Can you work these out from the model? Positions are in its coordinate system, mm. Give positions to 0.01 mm unless a question says otherwise; leave off trailing zeros. Order: outer loops, then holes, each group sorted by start corner. A loop starts at its lowest first (then second) coordinate and runs counter-clockwise, first axis right, second up. Notation, with made-up numbers: (7.25, -32.5) - (44.25, -32.5) arc R28 ccw to (44.25, -8.5) - close; hole circle Ø7 at (-30.75, 63). An arc over 180 degrees is marked (long way). Answer as CSV lines item,"result".
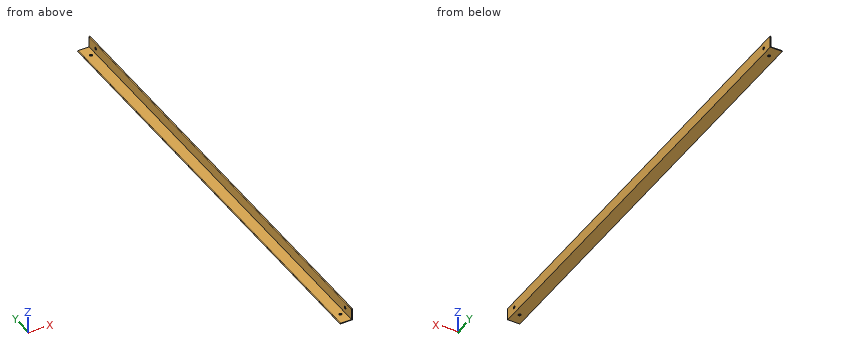
```python
from build123d import *

# Parameters (mm, degrees)
EXTRUDE_1_DEPTH        = 2000
FILLET_1_R             = 0.1
SKETCH_2_R             = 6
CUT_EXTRUDE_1_DEPTH    = 200
SKETCH_5_R             = 6
CUT_EXTRUDE_2_DEPTH    = 200
PATTERN_LINEAR_1_COUNT = 2
PATTERN_LINEAR_1_PITCH = 1900


with BuildPart() as part:
    # 草图1 → 凸台-拉伸1 (new body)
    with BuildSketch(Plane(origin=(0, 0, 0), x_dir=(1, 0, 0), z_dir=(0, 1, 0))):
        with BuildLine():
            ThreePointArc((-29.759542218, 3), (-28.958115236, 0.95539927), (-26.980771162, 0))
            Line((-26.980771162, 0), (-26.520700364, 0))
            Line((-26.520700364, 0), (20.240457782, 0))
            Line((20.240457782, 0), (20.240457782, -46.555391571))
            ThreePointArc((20.240457782, -46.555391571), (21.249360232, -48.99109755), (23.68506621, -50))
            Line((23.68506621, -50), (23.68506621, 3))
            Line((23.68506621, 3), (-29.759542218, 3))
        make_face()
    extrude(amount=EXTRUDE_1_DEPTH)

    # 圆角1
    # the kernel refuses this fillet: 0.1 mm, written as the material it takes off along each edge
    with BuildSketch(Plane(origin=(24.28506621, 2000, -3), x_dir=(0, 0, 1), z_dir=(-1, 0, 0))) as fillet_1_piece_1:
        with BuildLine():
            CenterArc((FILLET_1_R, -FILLET_1_R), FILLET_1_R, 90, 90)
            Line((0, -FILLET_1_R), (-FILLET_1_R * 0.02, -FILLET_1_R))
            Line((-FILLET_1_R * 0.02, -FILLET_1_R), (-FILLET_1_R * 0.02, FILLET_1_R * 0.0199999999995))
            Line((-FILLET_1_R * 0.02, FILLET_1_R * 0.0199999999995), (FILLET_1_R, FILLET_1_R * 0.0199999999995))
            Line((FILLET_1_R, FILLET_1_R * 0.0199999999995), (FILLET_1_R, 0))
        make_face()
    extrude(amount=54.644608429, mode=Mode.SUBTRACT)
    with BuildSketch(Plane(origin=(20.240457782, 2000, 0), x_dir=(0, 0, -1), z_dir=(-1, 0, 0)), Plane(origin=(-27.580771162, 0, 0), x_dir=(0, 0, -1), z_dir=(1, 0, 0))) as fillet_1_piece_2:
        with BuildLine():
            CenterArc((FILLET_1_R, FILLET_1_R), FILLET_1_R, 180, 90)
            Line((0, FILLET_1_R), (-FILLET_1_R * 0.02, FILLET_1_R))
            Line((-FILLET_1_R * 0.02, FILLET_1_R), (-FILLET_1_R * 0.02, -FILLET_1_R * 0.0199999999995))
            Line((-FILLET_1_R * 0.02, -FILLET_1_R * 0.0199999999995), (FILLET_1_R, -FILLET_1_R * 0.0199999999995))
            Line((FILLET_1_R, -FILLET_1_R * 0.0199999999995), (FILLET_1_R, 0))
        make_face()
    extrude(amount=47.821228944, mode=Mode.SUBTRACT)
    with BuildSketch(Plane(origin=(20.240457782, 2000, 0), x_dir=(1, 0, 0), z_dir=(0, 0, 1)), Plane(origin=(20.240457782, 0, 0), x_dir=(0, 1, 0), z_dir=(0, 0, 1))) as fillet_1_piece_3:
        with BuildLine():
            CenterArc((FILLET_1_R, -FILLET_1_R), FILLET_1_R, 90, 90)
            Line((0, -FILLET_1_R), (-FILLET_1_R * 0.02, -FILLET_1_R))
            Line((-FILLET_1_R * 0.02, -FILLET_1_R), (-FILLET_1_R * 0.02, FILLET_1_R * 0.0199999999995))
            Line((-FILLET_1_R * 0.02, FILLET_1_R * 0.0199999999995), (FILLET_1_R, FILLET_1_R * 0.0199999999995))
            Line((FILLET_1_R, FILLET_1_R * 0.0199999999995), (FILLET_1_R, 0))
        make_face()
    extrude(amount=46.555391571, mode=Mode.SUBTRACT)
    with BuildSketch(Plane(origin=(23.68506621, 2000, 46.555391571), x_dir=(-1, 0, 0), z_dir=(0, 0, -1))) as fillet_1_piece_4:
        with BuildLine():
            CenterArc((3.444608429 - FILLET_1_R, -FILLET_1_R), FILLET_1_R, 0, 90)
            Line((3.444608429, -FILLET_1_R), (3.444608429 + FILLET_1_R * 0.02, -FILLET_1_R))
            Line((3.444608429 + FILLET_1_R * 0.02, -FILLET_1_R), (3.444608429 + FILLET_1_R * 0.02, FILLET_1_R * 0.0199999999995))
            Line((3.444608429 + FILLET_1_R * 0.02, FILLET_1_R * 0.0199999999995), (3.444608429 - FILLET_1_R, FILLET_1_R * 0.0199999999995))
            Line((3.444608429 - FILLET_1_R, FILLET_1_R * 0.0199999999995), (3.444608429 - FILLET_1_R, 0))
        make_face()
    revolve(axis=Axis((23.68506621, 2000, 46.555391571), (0, 1, 0)), revolution_arc=99.984089086, mode=Mode.SUBTRACT)
    with BuildSketch(Plane(origin=(24.28506621, 0, -3), x_dir=(0, 0, 1), z_dir=(-1, 0, 0))) as fillet_1_piece_5:
        with BuildLine():
            CenterArc((FILLET_1_R, FILLET_1_R), FILLET_1_R, 180, 90)
            Line((0, FILLET_1_R), (-FILLET_1_R * 0.02, FILLET_1_R))
            Line((-FILLET_1_R * 0.02, FILLET_1_R), (-FILLET_1_R * 0.02, -FILLET_1_R * 0.02))
            Line((-FILLET_1_R * 0.02, -FILLET_1_R * 0.02), (FILLET_1_R, -FILLET_1_R * 0.02))
            Line((FILLET_1_R, -FILLET_1_R * 0.02), (FILLET_1_R, 0))
        make_face()
    extrude(amount=54.644608429, mode=Mode.SUBTRACT)
    with BuildSketch(Plane(origin=(23.68506621, 2000, 50.6), x_dir=(-1, 0, 0), z_dir=(0, 0, -1)), Plane(origin=(23.68506621, 0, 50.6), x_dir=(0, 1, 0), z_dir=(0, 0, -1))) as fillet_1_piece_6:
        with BuildLine():
            CenterArc((FILLET_1_R, -FILLET_1_R), FILLET_1_R, 90, 90)
            Line((0, -FILLET_1_R), (-FILLET_1_R * 0.02, -FILLET_1_R))
            Line((-FILLET_1_R * 0.02, -FILLET_1_R), (-FILLET_1_R * 0.02, FILLET_1_R * 0.0199999999995))
            Line((-FILLET_1_R * 0.02, FILLET_1_R * 0.0199999999995), (FILLET_1_R, FILLET_1_R * 0.0199999999995))
            Line((FILLET_1_R, FILLET_1_R * 0.0199999999995), (FILLET_1_R, 0))
        make_face()
    extrude(amount=54.2, mode=Mode.SUBTRACT)
    with BuildSketch(Plane(origin=(23.68506621, 0, 46.555391571), x_dir=(-1, 0, 0), z_dir=(0, 0, -1))) as fillet_1_piece_7:
        with BuildLine():
            CenterArc((3.444608429 - FILLET_1_R, FILLET_1_R), FILLET_1_R, 270, 90)
            Line((3.444608429 - FILLET_1_R, 0), (3.444608429 - FILLET_1_R, -FILLET_1_R * 0.02))
            Line((3.444608429 - FILLET_1_R, -FILLET_1_R * 0.02), (3.444608429 + FILLET_1_R * 0.02, -FILLET_1_R * 0.02))
            Line((3.444608429 + FILLET_1_R * 0.02, -FILLET_1_R * 0.02), (3.444608429 + FILLET_1_R * 0.02, FILLET_1_R))
            Line((3.444608429 + FILLET_1_R * 0.02, FILLET_1_R), (3.444608429, FILLET_1_R))
        make_face()
    revolve(axis=Axis((23.68506621, 0, 46.555391571), (0, 1, 0)), revolution_arc=99.984089086, mode=Mode.SUBTRACT)
    with BuildSketch(Plane(origin=(20.840457782, 2000, 0), x_dir=(0, 0, -1), z_dir=(-1, 0, 0))) as fillet_1_piece_8a_section:
        with BuildLine():
            CenterArc((FILLET_1_R, FILLET_1_R), FILLET_1_R, 180, 90)
            Line((0, FILLET_1_R), (-FILLET_1_R * 0.02, FILLET_1_R))
            Line((-FILLET_1_R * 0.02, FILLET_1_R), (-FILLET_1_R * 0.02, -FILLET_1_R * 0.0199999999995))
            Line((-FILLET_1_R * 0.02, -FILLET_1_R * 0.0199999999995), (FILLET_1_R, -FILLET_1_R * 0.0199999999995))
            Line((FILLET_1_R, -FILLET_1_R * 0.0199999999995), (FILLET_1_R, 0))
        make_face()
    fillet_1_piece_8a = extrude(amount=48.421228944, mode=Mode.PRIVATE)
    fillet_1_piece_8a = split(fillet_1_piece_8a, bisect_by=Plane(origin=(20.240457782, 1999.977360489, -0.022639511), z_dir=(1, 0, 0)), keep=Keep.TOP, mode=Mode.PRIVATE)
    with BuildSketch(Plane(origin=(20.240457782, 2000, -0.6), x_dir=(1, 0, 0), z_dir=(0, 0, 1))) as fillet_1_piece_8b_section:
        with BuildLine():
            CenterArc((FILLET_1_R, -FILLET_1_R), FILLET_1_R, 90, 90)
            Line((0, -FILLET_1_R), (-FILLET_1_R * 0.02, -FILLET_1_R))
            Line((-FILLET_1_R * 0.02, -FILLET_1_R), (-FILLET_1_R * 0.02, FILLET_1_R * 0.0199999999995))
            Line((-FILLET_1_R * 0.02, FILLET_1_R * 0.0199999999995), (FILLET_1_R, FILLET_1_R * 0.0199999999995))
            Line((FILLET_1_R, FILLET_1_R * 0.0199999999995), (FILLET_1_R, 0))
        make_face()
    fillet_1_piece_8b = extrude(amount=47.155391571, mode=Mode.PRIVATE)
    fillet_1_piece_8b = split(fillet_1_piece_8b, bisect_by=Plane(origin=(20.263097293, 1999.977360489, 0), z_dir=(0, 0, -1)), keep=Keep.TOP, mode=Mode.PRIVATE)
    fillet_1_piece_8 = fillet_1_piece_8a & fillet_1_piece_8b
    add(fillet_1_piece_8, mode=Mode.SUBTRACT)
    with BuildSketch(Plane(origin=(20.240457782, 0, -0.6), x_dir=(0, 1, 0), z_dir=(0, 0, 1))) as fillet_1_piece_9a_section:
        with BuildLine():
            CenterArc((FILLET_1_R, -FILLET_1_R), FILLET_1_R, 90, 90)
            Line((0, -FILLET_1_R), (-FILLET_1_R * 0.02, -FILLET_1_R))
            Line((-FILLET_1_R * 0.02, -FILLET_1_R), (-FILLET_1_R * 0.02, FILLET_1_R * 0.02))
            Line((-FILLET_1_R * 0.02, FILLET_1_R * 0.02), (FILLET_1_R, FILLET_1_R * 0.02))
            Line((FILLET_1_R, FILLET_1_R * 0.02), (FILLET_1_R, 0))
        make_face()
    fillet_1_piece_9a = extrude(amount=47.155391571, mode=Mode.PRIVATE)
    fillet_1_piece_9a = split(fillet_1_piece_9a, bisect_by=Plane(origin=(20.263097293, 0.022639511, 0), z_dir=(0, 0, -1)), keep=Keep.TOP, mode=Mode.PRIVATE)
    with BuildSketch(Plane(origin=(-27.580771162, 0, 0), x_dir=(0, 0, -1), z_dir=(1, 0, 0))) as fillet_1_piece_9b_section:
        with BuildLine():
            CenterArc((FILLET_1_R, FILLET_1_R), FILLET_1_R, 180, 90)
            Line((0, FILLET_1_R), (-FILLET_1_R * 0.02, FILLET_1_R))
            Line((-FILLET_1_R * 0.02, FILLET_1_R), (-FILLET_1_R * 0.02, -FILLET_1_R * 0.02))
            Line((-FILLET_1_R * 0.02, -FILLET_1_R * 0.02), (FILLET_1_R, -FILLET_1_R * 0.02))
            Line((FILLET_1_R, -FILLET_1_R * 0.02), (FILLET_1_R, 0))
        make_face()
    fillet_1_piece_9b = extrude(amount=48.421228944, mode=Mode.PRIVATE)
    fillet_1_piece_9b = split(fillet_1_piece_9b, bisect_by=Plane(origin=(20.240457782, 0.022639511, -0.022639511), z_dir=(1, 0, 0)), keep=Keep.TOP, mode=Mode.PRIVATE)
    fillet_1_piece_9 = fillet_1_piece_9a & fillet_1_piece_9b
    add(fillet_1_piece_9, mode=Mode.SUBTRACT)

    # 草图2 → 切除-拉伸1 (cut)
    with BuildSketch(Plane(origin=(23.68506621, 0, 0), x_dir=(0, 0, -1), z_dir=(1, 0, 0))):
        with Locations((-23.5, 50.1)):
            Circle(SKETCH_2_R)
        with Locations((-23.5, 1949.9)):
            Circle(SKETCH_2_R)
    extrude(amount=-CUT_EXTRUDE_1_DEPTH, mode=Mode.SUBTRACT)

    # 草图5 → 切除-拉伸2 (cut)
    with BuildSketch(Plane(origin=(0, 0, -3), x_dir=(-1, 0, 0), z_dir=(0, 0, -1))):
        with Locations((0, 50)):
            Circle(SKETCH_5_R)
    cut_extrude_2 = extrude(amount=-CUT_EXTRUDE_2_DEPTH, mode=Mode.SUBTRACT)

    # 阵列(线性)1: 切除-拉伸2 ×2
    with Locations(*[(0, i * PATTERN_LINEAR_1_PITCH, 0) for i in range(1, PATTERN_LINEAR_1_COUNT)]):
        add(cut_extrude_2, mode=Mode.SUBTRACT)


solid = part.part
```
1) I want a section at C-C on z = 8. Write out the boundary of the cut face in (x, y).
Answer block:
outline,"(20.24, 0.1) arc R0.1 ccw to (20.34, 0) - (23.59, 0) arc R0.1 ccw to (23.69, 0.1) - (23.69, 1999.9) arc R0.1 ccw to (23.59, 2000) - (20.34, 2000) arc R0.1 ccw to (20.24, 1999.9) - close"
2) I'm going to push flat-ended pins straight in: P1, Ø2, axis at y = 509, z = 11.5, coming from the -X side; P2, Ø10, axis at x = -7, y = 230.5, coming from the +Z side; P3, Ø19, axis at x = 0, y = 50, coming from the -Z side. Where does each tip first touch, or does it pass through?
Answer block:
P1,"x = 20.24"
P2,"z = 0"
P3,"z = -3"
3) I need wall thicknesses on line 1 along Y through (x, z) = (22, 23.5); line 2 along X through (y, z) = (1445.5, 37.5); line 3 along Z through (x, y) = (10, 1079). Which ranges of each line are inside material? Lowest first, please. Write a range as [from, to].
Answer block:
line 1,"[0, 44.1], [56.1, 1943.9], [1955.9, 2000]"
line 2,"[20.24, 23.69]"
line 3,"[-3, 0]"
4) I want a section at A-A on y = 1495.5. Write out the boundary of the cut face in (x, z), plus the area to 3 significant figures.
Answer block:
outline,"(-29.76, -3) - (23.69, -3) - (23.69, 50) arc R3.44 ccw to (20.24, 46.56) - (20.24, 0) - (-26.98, 0) arc R3.01 ccw to start"
area,"328 mm2"
5) I want a section at B-B on x = -16.5. Write out the boundary of the cut face in (y, z), plus the area to 3 significant figures.
Answer block:
outline,"(0, -2.9) arc R0.1 ccw to (0.1, -3) - (1999.9, -3) arc R0.1 ccw to (2000, -2.9) - (2000, -0.1) arc R0.1 ccw to (1999.9, 0) - (0.1, 0) arc R0.1 ccw to (0, -0.1) - close"
area,"6,000 mm2"
